Autodesk Inventor part; units mm, degrees
ref_plane "YZ Plane" through (0, 0, 0) normal (1, 0, 0) x (0, 1, 0)
ref_plane "XZ Plane" through (0, 0, 0) normal (0, 1, 0) x (-1, 0, 0)
ref_plane "XY Plane" through (0, 0, 0) normal (0, 0, 1) x (1, 0, 0)
sketch "Sketch1" plane through (0, 0, 0) normal (1, 0, 0) x (0, 1, 0)
  line L0 (6.5194, -26.4952) -> (6.5, 25.5048)
  line L1 (6.5, 25.5048) -> (-6.5, 25.5)
  line L2 (-6.5, 25.5) -> (-6.4806, -26.5)
  line L3 (-6.4806, -26.5) -> (6.5, 25.5048) construction
  line L4 (6.5194, -26.4952) -> (-6.5, 25.5) construction
  circle A0 centre (-0.0034, 14.5024) radius 1.25
  arc A1 (-6.4806, -26.5) -> (6.5194, -26.4952) centre (0.0194, -26.4976) ccw
  circle A2 centre (-0.0017, 22.0024) radius 1.25
  dimension "d8" = 13
  dimension "d12" = 2.5
  dimension "d22" = 52
  dimension "d23" = 6.5
  dimension "d24" = 90
  dimension "d25" = 90
  dimension "d26" = 11
  dimension "d27" = 2.5
  dimension "d28" = 7.5
extrude "Extrusion1" add sketch "Sketch1" along normal blind 8
sketch "Sketch2" plane through (0, 0, 0) normal (-1, 0, 0) x (0, 0, 1)
  arc A0 (-26.4952, 6.5194) -> (-26.5, -6.4806) centre (-26.4976, 0.0194) ccw
  circle A1 centre (-26.4976, 0.0194) radius 1.5
  point P0 (0, 0)
  dimension "d16" = 3
extrude "Extrusion2" add sketch "Sketch2" along normal blind 3
sketch "Sketch3" plane through (-3, 0.0194, -26.4976) normal (-1, 0, 0) x (0, 0, 1)
  circle A0 centre (0, 0) radius 1.5
  circle A1 centre (0, 0) radius 2.5
  point P0 (26.4976, -0.0194)
  dimension "d19" = 5
extrude "Extrusion3" add sketch "Sketch3" along normal blind 1.5 contours A0 | A1
properties part number "Arm2"
The listing builds one solid part. Answer for the finished solid, in the listing's coordinates (mm). A direction names the side the tool comes from. Round coordinates to 2 decimals unless told otherwise and drop trailing zeros. Order: outer loops, then holes, each group sorted by start corner. A loop starts at its lowest first (then second) coordinate and runs counter-clockwise, first axis right, second up. Notation, with made-up numbers: (-4.5, 22.25) -> (23.5, 22.25) arc R22 cw to (23.5, 40.25) -> close; hole circle Ø11 at (19, -39.75). An arc over 180 degrees is marked (long way). Write each question's results on one line, items separated by ' | '. Start each with the question number.
Q1. Straight lines are drawn through the part: probe 1 along X at (y, z) = (-5.75, -12.5); probe 2 along Y at (x, z) = (4, -1.5); probe 3 along Z at (x, y) = (3.75, 5.75). For each, find the intervals that lie inside material, in ascending order. Write a range as from..to.
Q2. Each of these flat-tipped pins is pushed along its axis until it touches: pin 1 (2 mm diameter, centred on y = 0, z = 14.5, fed in from +X); pin 2 (1.5 mm diameter, centred on x = 6, y = -1, fed in from -Z); pin 3 (4 mm diameter, centred on x = 1, z = -18, fed in from -Y); pin 4 (4 mm diameter, centred on x = 5, z = 2, fed in from +Y). Where does it stop, or does it pass through?
Q3. Find section A-A (z = 21.5). Determine the outline of the cut face in (x, y).
Q4. Find section B-B (x = 4.25). Determine the outline of the cut face in (y, z).
Q5. Find section C-C (y = -4.5). Determine the outline of the cut face in (x, z).
Q6. Find section D-D (z = -15). Determine the outline of the cut face in (x, y).
Q7. The mould has two halves that part along Z. Classify faces 1 (the flat face through (8, 0, -3)), 2 (the cylindrical face through (3.944, -0.273, 23.223)), 3 (the cylindrical face through (-3.74, -1.67, -28.34)): pulls with the +Z half, pulls with the -Z half, needs draft (parallel to the pull), parting line crosses it, or undercut.
Q8. Which of the six approach directions +Z, -Z, +X, -X, +Y, -Y give full straight-line access (tool end or side, diameter ignored) to faces 4 (the flat face through (-3, -1, -25)), 5 (the cylindrical face through (3.944, 0.573, 15.611))?
Worked answers:
1) probe 1: x = 0..8 | probe 2: y = -6.49..6.51 | probe 3: z = -29.57..25.5
2) pin 1: passes through | pin 2: stops at z = -32.99 | pin 3: stops at y = -6.48 | pin 4: stops at y = 6.51
3) outline: (0, -6.5) -> (8, -6.5) -> (8, -1.15) -> (0, -1.15) -> close; (0, 1.14) -> (8, 1.14) -> (8, 6.5) -> (0, 6.5) -> close
4) outline: (-6.5, 25.5) -> (-6.48, -26.5) arc R6.5 ccw to (6.52, -26.5) -> (6.5, 25.5) -> close; hole circle Ø2.5 at (0, 14.5); hole circle Ø2.5 at (0, 22)
5) outline: (0, -31.17) -> (8, -31.17) -> (8, 25.5) -> (0, 25.5) -> close
6) outline: (0, -6.48) -> (8, -6.48) -> (8, 6.52) -> (0, 6.52) -> close
7) face 1: needs draft | face 2: undercut | face 3: parting line crosses it
8) face 4: none | face 5: +X, -X
